```python
from build123d import *

# Parameters (mm, degrees)
SKETCH1_W           = 262.89
SKETCH1_H           = 317.5
BOSS_EXTRUDE1_DEPTH = 6.35
SKETCH2_W           = 82.55
SKETCH2_H           = 114.3
SKETCH2_R           = 8.128
CUT_EXTRUDE2_DEPTH  = 6.35
SKETCH2_5_R         = 8.128
CUT_EXTRUDE4_DEPTH  = 207.202989855


with BuildPart() as part:
    # Sketch1 → Boss-Extrude1 (new body)
    with BuildSketch(Plane.XY):
        Rectangle(SKETCH1_W, SKETCH1_H)
    extrude(amount=BOSS_EXTRUDE1_DEPTH)

    # Sketch2 → Cut-Extrude2 (cut)
    with BuildSketch(Plane.XY.offset(6.35)):
        with BuildLine():
            Line((47.625, -138.43), (47.625, -139.7))
            Line((47.625, -139.7), (47.625, -140.97))
            ThreePointArc((47.625, -140.97), (50.8, -144.145), (53.975, -140.97))
            Line((53.975, -140.97), (53.975, -138.43))
            ThreePointArc((53.975, -138.43), (50.8, -135.255), (47.625, -138.43))
        make_face()
        with BuildLine():
            Line((41.275, -140.97), (41.275, -139.7))
            Line((41.275, -139.7), (41.275, -138.43))
            ThreePointArc((41.275, -138.43), (38.1, -135.255), (34.925, -138.43))
            Line((34.925, -138.43), (34.925, -140.97))
            ThreePointArc((34.925, -140.97), (38.1, -144.145), (41.275, -140.97))
        make_face()
        with BuildLine():
            Line((-53.975, -100.33), (-53.975, -102.87))
            ThreePointArc((-53.975, -102.87), (-50.8, -106.045), (-47.625, -102.87))
            Line((-47.625, -102.87), (-47.625, -100.33))
            ThreePointArc((-47.625, -100.33), (-50.8, -97.155), (-53.975, -100.33))
        make_face()
        with BuildLine():
            ThreePointArc((-41.275, -102.87), (-38.1, -106.045), (-34.925, -102.87))
            Line((-34.925, -102.87), (-34.925, -100.33))
            ThreePointArc((-34.925, -100.33), (-38.1, -97.155), (-41.275, -100.33))
            Line((-41.275, -100.33), (-41.275, -102.87))
        make_face()
        with BuildLine():
            Line((-34.925, -140.97), (-34.925, -138.43))
            ThreePointArc((-34.925, -138.43), (-38.1, -135.255), (-41.275, -138.43))
            Line((-41.275, -138.43), (-41.275, -140.97))
            ThreePointArc((-41.275, -140.97), (-38.1, -144.145), (-34.925, -140.97))
        make_face()
        with BuildLine():
            ThreePointArc((-47.625, -138.43), (-50.8, -135.255), (-53.975, -138.43))
            Line((-53.975, -138.43), (-53.975, -140.97))
            ThreePointArc((-53.975, -140.97), (-50.8, -144.145), (-47.625, -140.97))
            Line((-47.625, -140.97), (-47.625, -138.43))
        make_face()
        with BuildLine():
            Line((34.925, -100.33), (34.925, -102.87))
            ThreePointArc((34.925, -102.87), (38.1, -106.045), (41.275, -102.87))
            Line((41.275, -102.87), (41.275, -100.33))
            ThreePointArc((41.275, -100.33), (38.1, -97.155), (34.925, -100.33))
        make_face()
        with BuildLine():
            ThreePointArc((47.625, -102.87), (50.8, -106.045), (53.975, -102.87))
            Line((53.975, -102.87), (53.975, -100.33))
            ThreePointArc((53.975, -100.33), (50.8, -97.155), (47.625, -100.33))
            Line((47.625, -100.33), (47.625, -102.87))
        make_face()
        with Locations((-44.45, 66.675)):
            Rectangle(SKETCH2_W, SKETCH2_H)
        with BuildLine():
            Line((-28.575, 135.255), (-28.575, 137.795))
            ThreePointArc((-28.575, 137.795), (-31.75, 140.97), (-34.925, 137.795))
            Line((-34.925, 137.795), (-34.925, 135.255))
            ThreePointArc((-34.925, 135.255), (-31.75, 132.08), (-28.575, 135.255))
        make_face()
        with BuildLine():
            ThreePointArc((-53.975, 137.795), (-57.15, 140.97), (-60.325, 137.795))
            Line((-60.325, 137.795), (-60.325, 135.255))
            ThreePointArc((-60.325, 135.255), (-57.15, 132.08), (-53.975, 135.255))
            Line((-53.975, 135.255), (-53.975, 137.795))
        make_face()
        with BuildLine():
            ThreePointArc((-34.925, -4.445), (-31.75, -7.62), (-28.575, -4.445))
            Line((-28.575, -4.445), (-28.575, -1.905))
            ThreePointArc((-28.575, -1.905), (-31.75, 1.27), (-34.925, -1.905))
            Line((-34.925, -1.905), (-34.925, -4.445))
        make_face()
        with BuildLine():
            Line((-60.325, -1.905), (-60.325, -4.445))
            ThreePointArc((-60.325, -4.445), (-57.15, -7.62), (-53.975, -4.445))
            Line((-53.975, -4.445), (-53.975, -1.905))
            ThreePointArc((-53.975, -1.905), (-57.15, 1.27), (-60.325, -1.905))
        make_face()
        with BuildLine():
            Line((28.575, -1.905), (28.575, -4.445))
            ThreePointArc((28.575, -4.445), (31.75, -7.62), (34.925, -4.445))
            Line((34.925, -4.445), (34.925, -1.905))
            ThreePointArc((34.925, -1.905), (31.75, 1.27), (28.575, -1.905))
        make_face()
        with BuildLine():
            ThreePointArc((53.975, -4.445), (57.15, -7.62), (60.325, -4.445))
            Line((60.325, -4.445), (60.325, -1.905))
            ThreePointArc((60.325, -1.905), (57.15, 1.27), (53.975, -1.905))
            Line((53.975, -1.905), (53.975, -4.445))
        make_face()
        with Locations((44.45, 66.675)):
            Rectangle(SKETCH2_W, SKETCH2_H)
        with BuildLine():
            ThreePointArc((34.925, 137.795), (31.75, 140.97), (28.575, 137.795))
            Line((28.575, 137.795), (28.575, 135.255))
            ThreePointArc((28.575, 135.255), (31.75, 132.08), (34.925, 135.255))
            Line((34.925, 135.255), (34.925, 137.795))
        make_face()
        with BuildLine():
            Line((60.325, 135.255), (60.325, 137.795))
            ThreePointArc((60.325, 137.795), (57.15, 140.97), (53.975, 137.795))
            Line((53.975, 137.795), (53.975, 135.255))
            ThreePointArc((53.975, 135.255), (57.15, 132.08), (60.325, 135.255))
        make_face()
        with Locations((-112.395, -57.15)):
            Circle(SKETCH2_R)
        with Locations((112.395, -57.15)):
            Circle(SKETCH2_R)
    extrude(amount=-CUT_EXTRUDE2_DEPTH, mode=Mode.SUBTRACT)

    # Sketch2<5> → Cut-Extrude4 (cut, through all)
    with BuildSketch(Plane.XY.offset(6.35)):
        with Locations((-112.395, 135.255)):
            Circle(SKETCH2_5_R)
        with Locations((112.395, 135.255)):
            Circle(SKETCH2_5_R)
    extrude(amount=-CUT_EXTRUDE4_DEPTH, mode=Mode.SUBTRACT)


solid = part.part
```
Part model, mm, in its own coordinate system. Round coordinates to 2 decimals unless told otherwise and drop trailing zeros. Write each loop counter-clockwise with the first axis right and the second up, starting at its lowest first coordinate (ties: lowest second). Pieces come first, ordered by that corner, then holes. Notation, with made-up numbers: (18, 27.5) -> (22, 27.5) arc R8 ccw to (22, 41.5) -> close; hole circle Ø7 at (55, 50.5). An arc over 180 degrees is marked (long way). Return JSON: item names as keys, results as strings. Group by question number.
Q1. Probe L1, parallel to X at y = 76, z = 1.5 (3 decimals); L2, parallel to Y at x = -66, z = 4.25 (3 decimals); L3, parallel to X at y = -98.5, z = 4.5 (3 decimals). List the from-to ranges inside material, lowest first. Write a range as [from, to].
Q2. Saw through at A-A on y = 116. Write the cut outline in (x, z) (3 decimals), plus the area to 3 significant figures.
Q3. Mould opens along Y. For faces 1 (the flat face through (-2, 2, 0)), 2 (the cylindrical face through (-38.17, -144.144, 3.219)) say: pulls with the +Y half, pulls with the -Y half, needs draft (parallel to the pull), parting line crosses it, or undercut.
Q4. Saw through at C-C on z = 4.5. State how many separate pieces and enclosed holes the cut face has, plus the area to 3 significant figures.
Q5. Pin check, flat tip, straight feed: pin 1 (3 mm diameter, centred on x = 105, y = 125, fed in from -Z). Stop position of the tip, or through.
Q6. Saw through at B-B on x = 115. Write the cut outline in (y, z), plus the area to 3 significant figures.
Answer:
{
 "1": {"L1": "[-131.445, -85.725], [-3.175, 3.175], [85.725, 131.445]", "L2": "[-158.75, 9.525], [123.825, 158.75]", "L3": "[-131.445, -53.395], [-48.205, -40.695], [-35.505, 35.505], [40.695, 48.205], [53.395, 131.445]"},
 "2": {"outline": "(-131.445, 0) -> (-85.725, 0) -> (-85.725, 6.35) -> (-131.445, 6.35) -> close; (-3.175, 0) -> (3.175, 0) -> (3.175, 6.35) -> (-3.175, 6.35) -> close; (85.725, 0) -> (131.445, 0) -> (131.445, 6.35) -> (85.725, 6.35) -> close", "area": "621 mm2"},
 "3": {"face 1": "needs draft", "face 2": "undercut"},
 "4": {"separate pieces": "1", "enclosed holes": "22", "area": "63,000 mm2"},
 "5": {"pin 1": "z = 0"},
 "6": {"outline": "(-158.75, 0) -> (-64.85, 0) -> (-64.85, 6.35) -> (-158.75, 6.35) -> close; (-49.45, 0) -> (127.56, 0) -> (127.56, 6.35) -> (-49.45, 6.35) -> close; (142.95, 0) -> (158.75, 0) -> (158.75, 6.35) -> (142.95, 6.35) -> close", "area": "1,820 mm2"}
}
